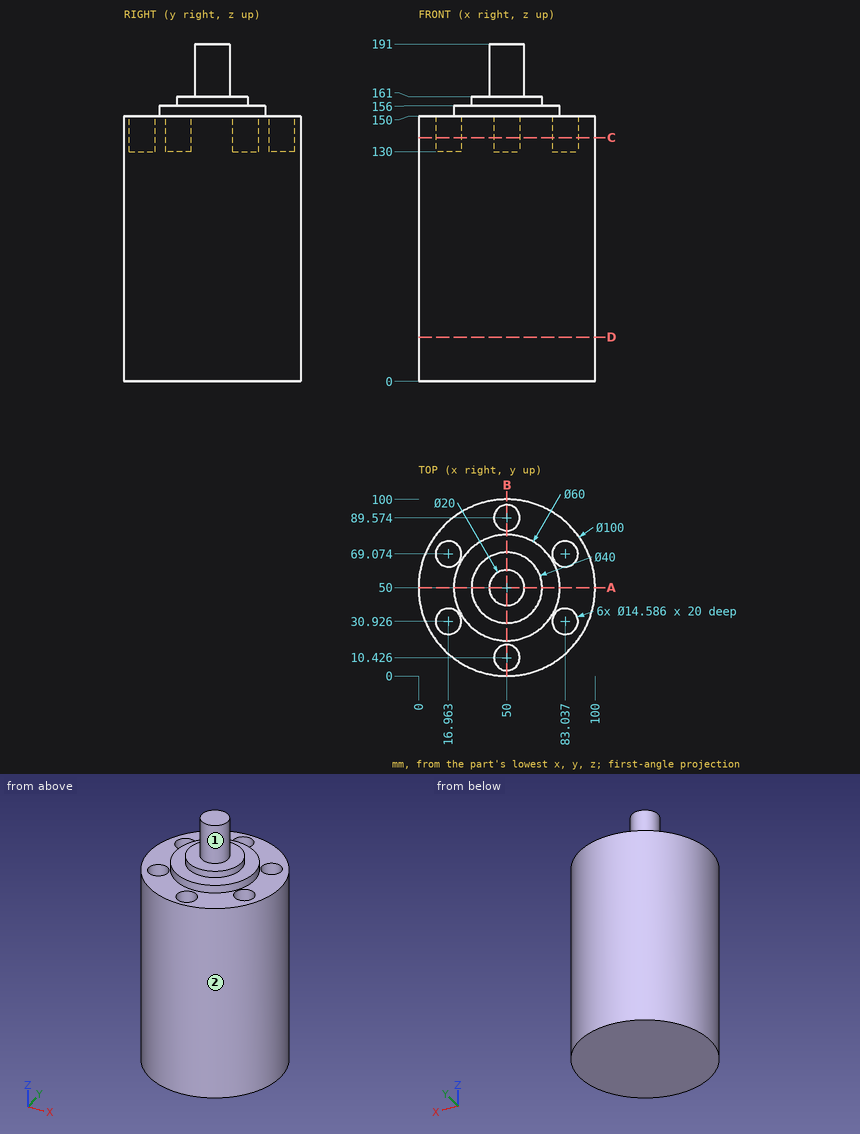
Geometry check sheet. Reference: drawing and pictorial views, mm from the part's lowest x, y, z. A direction names the side the tool comes from. Round coordinates to 2 decimals unless told otherwise and drop trailing zeros. Write each loop counter-clockwise with the first axis right and the second up, starting at its lowest first coordinate (ties: lowest second). Pieces come first, ordered by that corner, then holes.
Item 1: Material ranges on line 1 along X through (y, z) = (90, 148); line 2 along X through (y, z) = (34, 147); line 3 along Z through (x, y) = (25, 72), recorded low to high.
Determined:
line 1: x = 20 to 42.72, 57.28 to 80
line 2: x = 2.63 to 10.35, 23.58 to 76.42, 89.65 to 97.37
line 3: z = 0 to 150
Item 2: Section check D-D (z = 25). Record the boundary of the cut face in (x, y), plus the area to 3 significant figures.
Determined:
outline: circle Ø100 at (50, 50)
area: 7,850 mm2
Item 3: Section check C-C (z = 138). Record the boundary of the cut face in (x, y).
Determined:
outline: circle Ø100 at (50, 50); hole circle Ø14.59 at (16.96, 30.93); hole circle Ø14.59 at (16.96, 69.07); hole circle Ø14.59 at (50, 10.43); hole circle Ø14.59 at (50, 89.57); hole circle Ø14.59 at (83.04, 30.93); hole circle Ø14.59 at (83.04, 69.07)
Item 4: Section check B-B (x = 50). Record the boundary of the cut face in (y, z), plus the area to 3 significant figures.
Determined:
outline: (0, 0) - (100, 0) - (100, 150) - (96.87, 150) - (96.87, 130) - (82.28, 130) - (82.28, 150) - (80, 150) - (80, 156) - (70, 156) - (70, 161) - (60, 161) - (60, 191) - (40, 191) - (40, 161) - (30, 161) - (30, 156) - (20, 156) - (20, 150) - (17.72, 150) - (17.72, 130) - (3.13, 130) - (3.13, 150) - (0, 150) - close
area: 15,600 mm2
Item 5: Go/stop test with flat-tipped pins: pin 1 Ø11.5 at (x, y) = (83.04, 69.07) entering from +Z; pin 2 Ø16 at (x, y) = (81.5, 30.5) entering from +Z; pin 3 Ø10 at (y, z) = (14, 123.5) entering from -X. Record where each tip stops, or that it passes through.
Determined:
pin 1: stops at z = 130
pin 2: stops at z = 156
pin 3: stops at x = 10.77
Item 6: Section check A-A (y = 50). Record the boundary of the cut face in (x, z), plus the area to 3 significant figures.
Determined:
outline: (0, 0) - (100, 0) - (100, 150) - (80, 150) - (80, 156) - (70, 156) - (70, 161) - (60, 161) - (60, 191) - (40, 191) - (40, 161) - (30, 161) - (30, 156) - (20, 156) - (20, 150) - (0, 150) - close
area: 16,200 mm2
Item 7: Access from +Z, -Z, +X, -X, +Y, -Y to the whole of each face (thin tool, end or side, straight path). Record for the marked faces 1 and 2.
Determined:
face 1: +Z
face 2: +Z, -Z
